Geometry: see drawing. Coordinates: mm, zero at the bounding-box minimum. Give positions to 0.01 mm unless a question says otherwise; leave off trailing zeros. Order: outer loops, then holes, each group sorted by start corner. A loop starts at its lowest first (then second) coordinate and runs counter-clockwise, first axis right, second up. Notation, with made-up numbers: (-34.75, 67) - (-22.75, 67) arc R33 cw to (-22.75, 103) - close; hole circle Ø3 at (22, 29.25). An arc over 180 degrees is marked (long way). One line per item, written item: value.
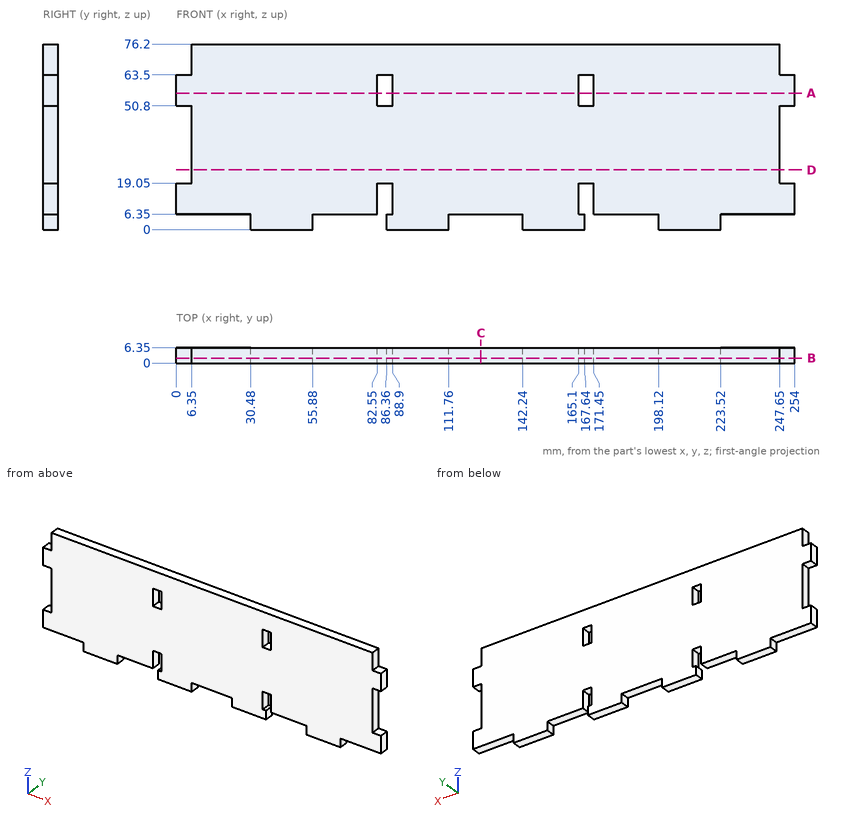
1) Material intervals for line 1 along X through (y, z) = (1, 16); line 2 along Z through (x, y) = (85, 3.5); line 3 along Z through (x, y) = (227.5, 4), sorted ascending.
Answers below:
line 1: 0 to 82.55, 88.9 to 165.1, 171.45 to 254
line 2: 19.05 to 50.8, 63.5 to 76.2
line 3: 6.35 to 76.2
2) First-contact query: pin 1 (3 mm diameter, centred on x = 132, y = 4.5, fed in from -Z); pin 2 (1.9 mm diameter, centred on y = 4.5, z = 3, fed in from -X); pin 3 (3 mm diameter, centred on y = 4.5, z = 4, fed in from +X); pin 4 (4 mm diameter, centred on x = 227, z = 39.5, fed in from -Y). Flat tips, straight axial feed; report the tip coordinate or a pass-through.
Answers below:
pin 1: z = 6.35
pin 2: x = 30.48
pin 3: x = 223.52
pin 4: y = 0
3) Section D-D, the plane z = 24.5. Return loops of the section in (x, y).
Answers below:
outline: (6.35, 0) - (247.65, 0) - (247.65, 6.35) - (6.35, 6.35) - close
4) Section A-A, the plane z = 56. Return loops of the section in (x, y).
Answers below:
outline: (0, 0) - (82.55, 0) - (82.55, 6.35) - (0, 6.35) - close; (88.9, 0) - (165.1, 0) - (165.1, 6.35) - (88.9, 6.35) - close; (171.45, 0) - (254, 0) - (254, 6.35) - (171.45, 6.35) - close
5) Section C-C, the plane x = 125. Return loops of the section in (y, z).
Answers below:
outline: (0, 6.35) - (6.35, 6.35) - (6.35, 76.2) - (0, 76.2) - close
6) Section B-B, the plane y = 2. Count the separate pieces of the cut face and the enclosed holes in it, then the cut area to 3 significant figures.
Answers below:
separate pieces: 1
enclosed holes: 2
area: 17,500 mm^2
